```python
from build123d import *

# Parameters (mm, degrees)
BOSS_EXTRUDE1_DEPTH = 300
FILLET1_R           = 1.5
SKETCH2_W           = 20
SKETCH2_H           = 300
CUT_EXTRUDE1_DEPTH  = 10
FILLET2_R           = 0.8


with BuildPart() as part:
    # Sketch1 → Boss-Extrude1 (new body)
    with BuildSketch(Plane.XY.offset(280)):
        Polygon((-7, 4), (4, -7), (7, -7), (7, -3), (20, -3), (20, 0), (0, 0), (0, 20), (-3, 20), (-3, 7), (-7, 7), align=None)
    extrude(amount=-BOSS_EXTRUDE1_DEPTH)

    # Fillet1
    fillet1_edges = [part.edges().sort_by_distance(p)[0] for p in [
        (4, -7, 130),
        (-7, 4, 130),
    ]]
    fillet(fillet1_edges, radius=FILLET1_R)

    # Sketch2 → Cut-Extrude1 (cut)
    with BuildSketch(Plane(origin=(0, 0, 0), x_dir=(1, 0, 0), z_dir=(0, 1, 0))):
        with Locations((10, -130)):
            Rectangle(SKETCH2_W, SKETCH2_H)
    extrude(amount=-CUT_EXTRUDE1_DEPTH, mode=Mode.SUBTRACT)

    # Fillet2
    fillet2_edges = [part.edges().sort_by_distance(p)[0] for p in [
        (0, -3, 130),
    ]]
    fillet(fillet2_edges, radius=FILLET2_R)


solid = part.part
```
Can you work these out from the model? Positions are in its coordinate system, mm. A direction names the side the tool comes from. Coordinates: 2 decimals unless noted, no trailing zeros. Write each loop counter-clockwise with the first axis right and the second up, starting at its lowest first coordinate (ties: lowest second). Pieces come first, ordered by that corner, then holes. Notation, with made-up numbers: (83, 22.25) - (141, 22.25) arc R14 cw to (141, 34.25) - close; hole circle Ø8 at (67.25, 21.5). An arc over 180 degrees is marked (long way). Return JSON: item names as keys, results as strings.
Q1. If we section it at B-B (x = -4.75): Please give me the cut outline in (y, z).
Computed values:
{"outline": "(1.75, -20) - (7, -20) - (7, 280) - (1.75, 280) - close"}
Q2. Please list where these lines run through material, in increasing order: L1, parallel to X at y = 11.25, z = 71.5; L2, parallel to Y at x = -1, z = 47; L3, parallel to X at y = 3.5, z = 34.5. Write a range as from..to.
Computed values:
{"L1": "x = -3..0", "L2": "y = -1.84..20", "L3": "x = -6.5..0"}
Q3. On a 3-axis mill with a long thin cutter (end or side, diameter ignored), from which of +Z, -Z, +X, -X, +Y, -Y can I reach the whole of each face in a straight line? I mean faces 1 (the flat face through (-3, 14, 132)), 2 (the flat face through (-2.8, 9.2, -20)). Say none if no direction works.
Computed values:
{"face 1": "+Z, -Z, -X, +Y", "face 2": "-Z, +X, -X, +Y, -Y"}
Q4. I'm going to push flat-ended pins straight in: pin 1 Ø6.5 at (y, z) = (11.5, 78) entering from -X; pin 2 Ø3 at (y, z) = (3, 114.5) entering from -X. Where does each tip first touch, or does it pass through?
Computed values:
{"pin 1": "stops at x = -3", "pin 2": "stops at x = -7"}
Q5. If we section it at A-A (z = 30.5): Please give me the cut outline in (x, y).
Computed values:
{"outline": "(-7, 4.62) arc R1.5 ccw to (-6.56, 3.56) - (-1.37, -1.63) arc R0.8 ccw to (0, -1.07) - (0, 20) - (-3, 20) - (-3, 7) - (-7, 7) - close"}
Q6. If we section it at C-C (y = 10.5): Please give me the cut outline in (x, z), then the cut area to 3 significant figures.
Computed values:
{"outline": "(-3, -20) - (0, -20) - (0, 280) - (-3, 280) - close", "area": "900 mm2"}
